Could you check a few things on this model? Use its own coordinates, in mm. Face numbers are marked on the shaded views. Round coordinates to 2 decimals unless told otherwise and drop trailing zeros. Write each loop counter-clockwise with the first axis right and the second up, starting at its lowest first coordinate (ties: lowest second). Pieces come first, ordered by that corner, then holes. Notation, with made-up numbers: (-31, 50) -> (1, 50) arc R21 ccw to (1, 89) -> close; hole circle Ø3 at (-9.5, 19.5). An arc over 180 degrees is marked (long way). Answer as CSV lines item,"result". Start each with the question number.
Q1. Imagine slicing it at D-D on y = 9. Give the number of separate pieces and of enclosed holes in the cut face, and give its area (3 significant figures).
Q2. If I drill on line 1 (X direction, y = 9.5, z = 41); line 2 (X direction, y = 2.25, z = -62); line 3 (X direction, y = 14.75, z = 1), over which ranges is the centre line in solid material (lowest first)? Write a range as [from, to].
Q3. Will these pins go through, and if not, where does the flat tip stop? pin 1 Ø3 at (y, z) = (9, 28) entering from -X; pin 2 Ø3.5 at (x, z) = (19.07, -62.14) entering from -Y; pin 3 Ø7 at (x, z) = (19.07, 70.41) entering from +Y.
Q4. Imagine slicing it at B-B on x = 2. Please give me the cut outline in (y, z).
Q5. Imagine slicing it at A-A on z = -41. Please give me the cut outline in (x, y), and give its area (3 significant figures).
Q6. Imagine slicing it at C-C on x = 18. Please give me the cut outline in (y, z).
Q7. If we mould it in two halves opening along X, with no side actions, what happens to the marked faces 1, 2 and 3? For each: pulls with the +X half, pulls with the -X half, needs draft (parallel to the pull), parting line crosses it, or undercut.
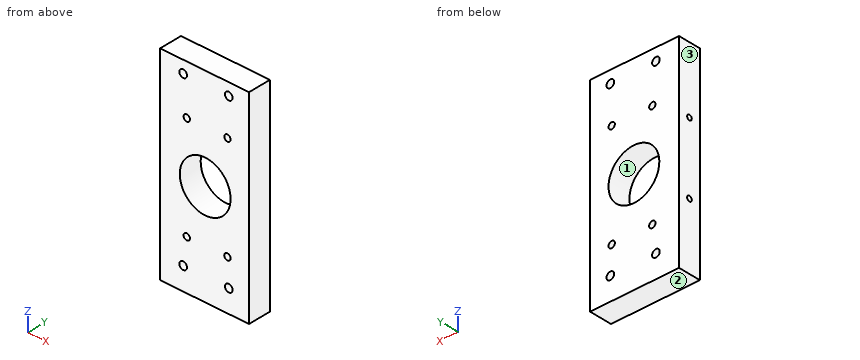
from build123d import *

# Parameters (mm, degrees)
SKETCH1_W                    = 70
SKETCH1_H                    = 160
BOSS_EXTRUDE1_DEPTH          = 18
SKETCH2_R                    = 20
CUT_EXTRUDE1_DEPTH           = 90.157164603
F_6_0_6_DIAMETER_HOLE1_D     = 6
F_4_0_4_DIAMETER_HOLE1_D     = 4
F_4_0_4_DIAMETER_HOLE1_DEPTH = 30
F_5_0_5_DIAMETER_HOLE1_D     = 5


with BuildPart() as part:
    # Sketch1 → Boss-Extrude1 (new body)
    with BuildSketch(Plane(origin=(0, 0, 0), x_dir=(1, 0, 0), z_dir=(0, 1, 0))):
        Rectangle(SKETCH1_W, SKETCH1_H)
    extrude(amount=BOSS_EXTRUDE1_DEPTH)

    # Sketch2 → Cut-Extrude1 (cut, through all)
    with BuildSketch(Plane(origin=(0, 18, 0), x_dir=(1, 0, 0), z_dir=(0, 1, 0))):
        with Locations(Location((0.500000036, 0.001841312, 0), (0, 0, 270))):
            Circle(SKETCH2_R)
    extrude(amount=-CUT_EXTRUDE1_DEPTH, mode=Mode.SUBTRACT)

    # Ø6.0 (6) Diameter Hole1 (through all)
    with Locations(Plane(origin=(0, 18, 0), x_dir=(1, 0, 0), z_dir=(0, 1, 0))):
        with Locations((19.069096126, 62.135567862), (-16.824568918, 62.135567862), (19.069096126, -70.412962857), (-16.824568918, -70.412962857)):
            Hole(F_6_0_6_DIAMETER_HOLE1_D / 2)

    # Ø4.0 (4) Diameter Hole1
    with Locations(Plane.ZY.offset(35)):
        with Locations((28, 9), (-28, 9)):
            Hole(F_4_0_4_DIAMETER_HOLE1_D / 2, depth=F_4_0_4_DIAMETER_HOLE1_DEPTH)

    # Ø5.0 (5) Diameter Hole1 (through all)
    with Locations(Plane(origin=(0, 18, 0), x_dir=(1, 0, 0), z_dir=(0, 1, 0))):
        with Locations((18, 41), (-14, 41), (18, -41), (-14, -41)):
            Hole(F_5_0_5_DIAMETER_HOLE1_D / 2)


solid = part.part
Checks:
1,separate pieces,"1"
1,enclosed holes,"9"
1,area,"9,510 mm^2"
2,line 1,"[-35, -16.5], [-11.5, 15.5], [20.5, 35]"
2,line 2,"[-35, -19.82], [-13.83, 16.07], [22.07, 35]"
2,line 3,"[-35, -19.47], [20.47, 35]"
3,pin 1,"x = -5"
3,pin 2,"through"
3,pin 3,"y = 18"
4,outline,"(0, -80) -> (18, -80) -> (18, -19.95) -> (0, -19.95) -> close; (0, 19.94) -> (18, 19.94) -> (18, 80) -> (0, 80) -> close"
5,outline,"(-35, 0) -> (-16.5, 0) -> (-16.5, 18) -> (-35, 18) -> close; (-11.5, 0) -> (15.5, 0) -> (15.5, 18) -> (-11.5, 18) -> close; (20.5, 0) -> (35, 0) -> (35, 18) -> (20.5, 18) -> close"
5,area,"1,080 mm^2"
6,outline,"(0, -80) -> (18, -80) -> (18, -64.94) -> (0, -64.94) -> close; (0, -59.33) -> (18, -59.33) -> (18, -43.5) -> (0, -43.5) -> close; (0, -38.5) -> (18, -38.5) -> (18, -9.68) -> (0, -9.68) -> close; (0, 9.68) -> (18, 9.68) -> (18, 38.5) -> (0, 38.5) -> close; (0, 43.5) -> (18, 43.5) -> (18, 67.61) -> (0, 67.61) -> close; (0, 73.22) -> (18, 73.22) -> (18, 80) -> (0, 80) -> close"
7,face 1,"undercut"
7,face 2,"needs draft"
7,face 3,"pulls with the -X half"
